Design review of the part built by this model. Coordinates are the model's own, in mm. Face numbers are marked on the shaded views. Round coordinates to 2 decimals unless told otherwise and drop trailing zeros. Order: outer loops, then holes, each group sorted by start corner. A loop starts at its lowest first (then second) coordinate and runs counter-clockwise, first axis right, second up. Notation, with made-up numbers: (61, -35) - (83, -35) arc R22 cw to (83, -16) - close; hole circle Ø4 at (47.25, -30). An arc over 180 degrees is marked (long way). Write item = value, one per line.
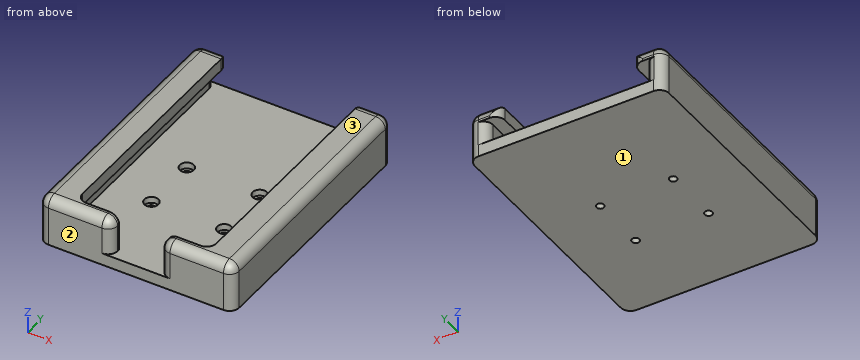
from build123d import *

# Parameters (mm, degrees)
F0_W          = 101.6
F0_H          = 127
F1_DEPTH      = 6.35
F2_W          = 9.525
F2_H          = 127
F3_DEPTH      = 12.7
F4_W          = 6.35
F4_H          = 127
F4_W_2        = 9.525
F4_W_3        = 15.875
F5_DEPTH      = 6.35
F6_R          = 3.683
F7_DEPTH      = 3.302
F8_R          = 1.9685
F9_DEPTH      = 25.4
F10_W         = 25.4
F10_H         = 6.35
F11_DEPTH     = 6.35
F12_R         = 5.08
F13_R         = 5.08
F14_T4_DEPTH  = 25.4
F14_T9_DEPTH  = 25.4
F14_T11_DEPTH = 12.7
F15_R         = 5.08


# Not quite as in the source:
# - a fillet or chamfer that OpenCascade refuses, or shapes differently, is made with other operations: its cross-section is extruded or revolved along the edge and cut away or added


with BuildPart() as f1:
    # F0 (on Top) → F1 (new body)
    with BuildSketch(Plane.XY):
        Rectangle(F0_W, F0_H)
    extrude(amount=F1_DEPTH)

    # F2 (on face) → F3 (join)
    with BuildSketch(Plane.XY.offset(6.35)):
        with Locations((-46.0375, 0)):
            Rectangle(F2_W, F2_H)
        with Locations((46.0375, 0)):
            Rectangle(F2_W, F2_H)
    extrude(amount=F3_DEPTH)

    # F4 (on face) → F5 (join)
    with BuildSketch(Plane.XY.offset(19.05)):
        with Locations((-38.1, 0)):
            Rectangle(F4_W, F4_H)
        with Locations((-46.0375, 0)):
            Rectangle(F4_W_2, F4_H)
        with Locations((42.8625, 0)):
            Rectangle(F4_W_3, F4_H)
    extrude(amount=F5_DEPTH)

    # F6 (on face) → F7 (cut)
    with BuildSketch(Plane.XY.offset(6.35)):
        with Locations((-19.05, 3.81)):
            Circle(F6_R)
        with Locations((-19.05, -26.035)):
            Circle(F6_R)
        with Locations((19.05, -26.035)):
            Circle(F6_R)
        with Locations((19.05, 3.81)):
            Circle(F6_R)
    extrude(amount=-F7_DEPTH, mode=Mode.SUBTRACT)

    # F8 (on face) → F9 (cut)
    with BuildSketch(Plane.XY.offset(3.048)):
        with Locations((-19.05, 3.81)):
            Circle(F8_R)
        with Locations((19.05, 3.81)):
            Circle(F8_R)
        with Locations((-19.05, -26.035)):
            Circle(F8_R)
        with Locations((19.05, -26.035)):
            Circle(F8_R)
    extrude(amount=-F9_DEPTH, mode=Mode.SUBTRACT)

    # F10 (on face) → F11 (join)
    with BuildSketch(Plane.XZ.offset(63.5)):
        Polygon((-34.925, 25.4), (-50.8, 25.4), (-50.8, 0), (-12.7, 0), (-12.7, 6.35), (-41.275, 6.35), (-41.275, 19.05), (-34.925, 19.05), align=None)
        Polygon((-12.7, 25.4), (-34.925, 25.4), (-34.925, 19.05), (-41.275, 19.05), (-41.275, 6.35), (-12.7, 6.35), align=None)
        Polygon((34.925, 25.4), (12.7, 25.4), (12.7, 6.35), (41.275, 6.35), (41.275, 19.05), (34.925, 19.05), align=None)
        Polygon((12.7, 6.35), (12.7, 0), (50.8, 0), (50.8, 25.4), (34.925, 25.4), (34.925, 19.05), (41.275, 19.05), (41.275, 6.35), align=None)
        with Locations((0, 3.175)):
            Rectangle(F10_W, F10_H)
    extrude(amount=F11_DEPTH)

    # F12
    f12_edges = [f1.edges().sort_by_distance(p)[0] for p in [
        (-50.8, -3.175, 25.4),
        (50.8, -3.175, 25.4),
    ]]
    fillet(f12_edges, radius=F12_R)

    # F13
    f13_edges = [f1.edges().sort_by_distance(p)[0] for p in [
        (-34.925, 63.5, 22.225),
        (34.925, 63.5, 22.225),
        (-50.8, 63.5, 10.16),
        (50.8, 63.5, 10.16),
        (-50.8, -69.85, 10.16),
        (50.8, -69.85, 10.16),
        (-34.925, -63.5, 22.225),
        (34.925, -63.5, 22.225),
    ]]
    fillet(f13_edges, radius=F13_R)

    # F14: fillet of radius 5.08 on 4 edges, made by hand


with BuildPart() as f14_tool2:
    # F14_s3 → F14_t4 (new body)
    with BuildSketch(Plane.XY.offset(6.35)):
        with BuildLine():
            ThreePointArc((-41.275, -58.42), (-39.7871024484, -62.0121024484), (-36.195, -63.5))
            Line((-36.195, -63.5), (-41.275, -63.5))
            Line((-41.275, -63.5), (-41.275, -58.42))
        make_face()
    extrude(amount=F14_T4_DEPTH)

    split(bisect_by=Plane.XY.offset(25.4), keep=Keep.BOTTOM)


with BuildPart() as f1_1:
    add(f1.part)

    # F14_t1: union F14_tool2
    add(f14_tool2.part)


with BuildPart() as f14_tool7:
    # F14_s8 → F14_t9 (new body)
    with BuildSketch(Plane.XY.offset(6.35)):
        with BuildLine():
            ThreePointArc((41.275, -58.42), (39.7871024484, -62.0121024484), (36.195, -63.5))
            Line((36.195, -63.5), (41.275, -63.5))
            Line((41.275, -63.5), (41.275, -58.42))
        make_face()
    extrude(amount=F14_T9_DEPTH)

    split(bisect_by=Plane.XY.offset(25.4), keep=Keep.BOTTOM)


with BuildPart() as f1_2:
    add(f1_1.part)

    # F14_t6: union F14_tool7
    add(f14_tool7.part)

    # F14_s12 → F14_t11 (cut)
    with BuildSketch(Plane.XY.offset(6.35)):
        with BuildLine():
            ThreePointArc((-46.355, 63.5), (-42.7628975516, 62.0121024484), (-41.275, 58.42))
            Line((-41.275, 58.42), (-41.275, 63.5))
            Line((-41.275, 63.5), (-46.355, 63.5))
        make_face()
        with BuildLine():
            ThreePointArc((46.355, 63.5), (42.7628975516, 62.0121024484), (41.275, 58.42))
            Line((41.275, 58.42), (41.275, 63.5))
            Line((41.275, 63.5), (46.355, 63.5))
        make_face()
    extrude(amount=F14_T11_DEPTH, mode=Mode.SUBTRACT)

    # F15
    f15_edges = [f1_2.edges().sort_by_distance(p)[0] for p in [
        (-12.7, -64.135, 25.4),
        (12.7, -64.135, 25.4),
        (-12.7, -69.85, 13.335),
        (12.7, -69.85, 13.335),
        (12.7, -68.362102, 23.912102),
        (-12.7, -68.362102, 23.912102),
    ]]
    fillet(f15_edges, radius=F15_R)


solid = f1_2.part
Item 1: Insertion check: P1, Ø8, axis at x = -20, y = -26, coming from the +Z side; P2, Ø3.5, axis at x = -19.5, y = 4.5, coming from the +Z side; P3, Ø1.5, axis at x = 31, y = -9, coming from the -Z side; P4, Ø5.5, axis at x = 29, z = 11.5, coming from the +Y side. Each pin has a flat end and moves straight along its axis. Give the tip position at first contact, or say it passes through.
Data:
P1 = 6.35
P2 = 3.05
P3 = 0
P4 = -63.5
Item 2: For line 1 along Y through (x, z) = (-19.05, 1.85); line 2 along X through (y, z) = (-18.5, 20.5) (3 decimals); line 3 along Z through (x, y) = (40.5, 47.5), list the stretches that pass through material, from the lowest coordinate up. Write a range as [from, to].
Data:
line_1 = [-69.85, -28], [-24.07, 1.84], [5.78, 63.5]
line_2 = [-50.797, -34.925], [34.925, 50.797]
line_3 = [0, 6.35], [19.05, 25.4]
Item 3: The part is to be moulded in two halves that separate along Z. For the marked faces 1, 2 and 3, say which applies: +Z half, -Z half, draft (parallel to the pull), parting line (faces both ways), or undercut.
Data:
face_1 = -Z half
face_2 = draft
face_3 = +Z half
Item 4: Take a section at D-D, the plane y = 48. State the section outline as (x, z) points (3 decimals).
Data:
outline = (-50.8, 0) - (50.8, 0) - (50.8, 20.32) arc R5.08 ccw to (45.72, 25.4) - (34.925, 25.4) - (34.925, 19.05) - (41.275, 19.05) - (41.275, 6.35) - (-41.275, 6.35) - (-41.275, 19.05) - (-34.925, 19.05) - (-34.925, 25.4) - (-45.72, 25.4) arc R5.08 ccw to (-50.8, 20.32) - close
Item 5: Take a section at C-C, the plane x = -9. State the section outline as (y, z) points.
Data:
outline = (-69.85, 0) - (63.5, 0) - (63.5, 6.35) - (-69.85, 6.35) - close
Item 6: Take a section at A-A, the plane y = 3.81. Count the separate pieces of the cut face and the enclosed holes in it, and give its area (3 significant figures).
Data:
separate_pieces = 3
enclosed_holes = 0
area = 1,000 mm2
